For this review, use the dimensioned drawing (mm, ordinates from the lowest corner) and the shaded views. A direction names the side the tool comes from. Round coordinates to 2 decimals unless told otherwise and drop trailing zeros. Write each loop counter-clockwise with the first axis right and the second up, starting at its lowest first coordinate (ties: lowest second). Pieces come first, ordered by that corner, then holes.
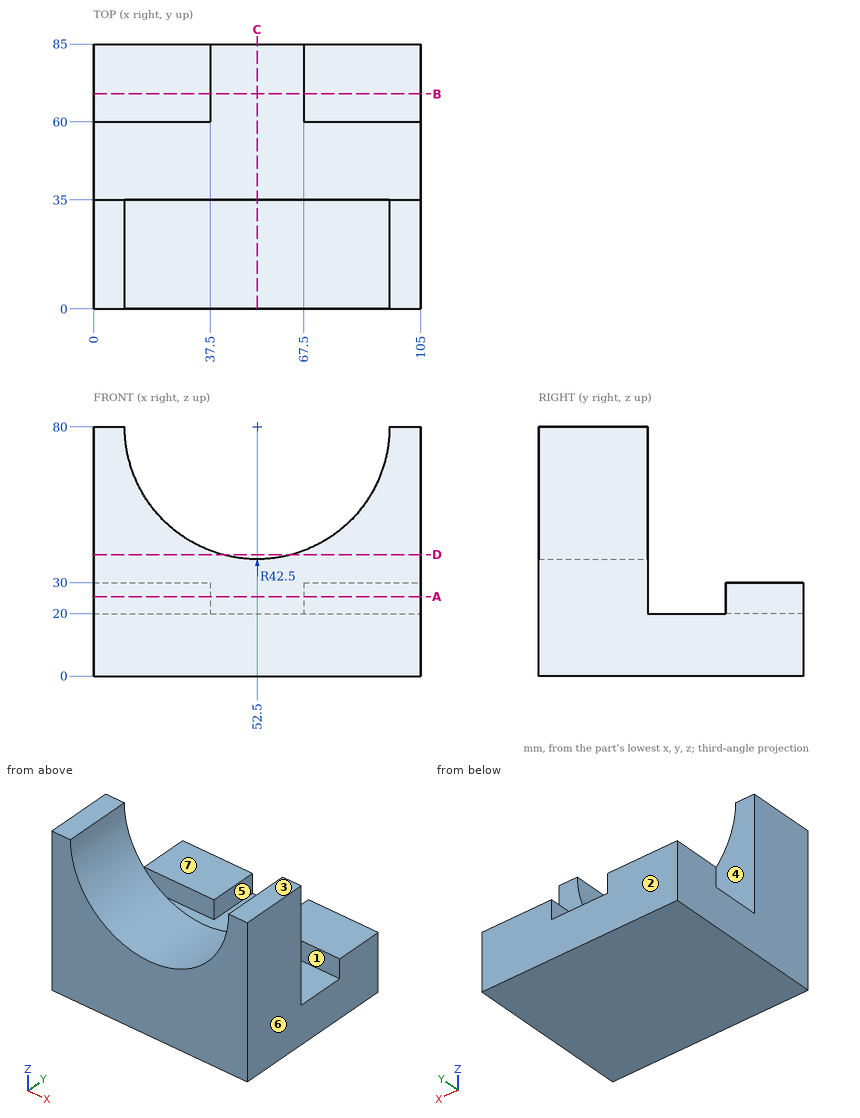
1) Add section B-B on y = 69. State the section outline as (x, z) points, and give its area (3 significant figures).
2) For the marked faces 4, 5, 6 and 7, list the 3-axis set-ups (+Z, -Z, +X, -X, +Y, -Y) from which the entire face can be reached by the end or side of a thin tool; tool diameter is ignored.
3) Add section D-D on z = 39. State the section outline as (x, y) points.
4) The part is to be moulded in two halves that separate along Y. For the marked faces 1, 2 and 3, say which applies: pulls with the +Y half, pulls with the -Y half, needs draft (parallel to the pull), parting line crosses it, or undercut.
5) For P1, Ø12.5, axis at x = 80.5, y = 70.5, coming from the +Z side; P2, Ø8, axis at x = 46, y = 40.5, coming from the +Z side; P3, Ø1, axis at x = 32.5, z = 37, coming from the +Y side, all flat-tipped, find the tip position at first contact; note any pin that passes through.
6) Add section A-A on z = 25.5. State the section outline as (x, y) points.
7) Add section C-C on x = 52.5. State the section outline as (y, z) points, and give its area (3 significant figures).
8) For line 1 along Y through (x, z) = (28.5, 29.5); line 2 along Z through (x, y) = (95, 44); line 3 along X through (y, z) = (76, 28.5), list the stretches that pass through material, from the lowest coordinate up.
Computed:
1. outline: (0, 0) - (105, 0) - (105, 30) - (67.5, 30) - (67.5, 20) - (37.5, 20) - (37.5, 30) - (0, 30) - close
1. area: 2,850 mm2
2. face 4: +Z, +X, -X
2. face 5: +Z, +Y
2. face 6: +Z, -Z, +X, +Y, -Y
2. face 7: +Z, +X, -X, +Y
3. outline: (0, 0) - (41.31, 0) - (41.31, 35) - (0, 35) - close; (63.69, 0) - (105, 0) - (105, 35) - (63.69, 35) - close
4. face 1: undercut
4. face 2: pulls with the +Y half
4. face 3: needs draft
5. P1: stops at z = 30
5. P2: stops at z = 20
5. P3: stops at y = 35
6. outline: (0, 0) - (105, 0) - (105, 35) - (0, 35) - close; (0, 60) - (37.5, 60) - (37.5, 85) - (0, 85) - close; (67.5, 60) - (105, 60) - (105, 85) - (67.5, 85) - close
7. outline: (0, 0) - (85, 0) - (85, 20) - (35, 20) - (35, 37.5) - (0, 37.5) - close
7. area: 2,310 mm2
8. line 1: y = 0 to 35, 60 to 85
8. line 2: z = 0 to 20
8. line 3: x = 0 to 37.5, 67.5 to 105
